```python
from build123d import *

# Parameters (mm, degrees)
SKETCH_2_R          = 2
EXTRUDE_1_DEPTH     = 44.1
CUT_EXTRUDE_START   = -7
CUT_EXTRUDE_1_DEPTH = 7
CHAMFER_1_SIZE      = 0.5
CHAMFER_2_SIZE      = 0.5


with BuildPart() as part:
    # Эскиз2 → Бобышка-Вытянуть1 (new body)
    with BuildSketch(Plane.XY):
        Circle(SKETCH_2_R)
    extrude(amount=EXTRUDE_1_DEPTH)

    # Эскиз3 → Вырез-Вытянуть1 (cut)
    with BuildSketch(Plane.XY.offset(44.1).offset(CUT_EXTRUDE_START)):
        with BuildLine():
            Line((1.322875656, 1.5), (-1.322875656, 1.5))
            ThreePointArc((-1.322875656, 1.5), (0, 2), (1.322875656, 1.5))
        make_face()
    extrude(amount=CUT_EXTRUDE_1_DEPTH, mode=Mode.SUBTRACT)

    # Фаска1
    chamfer_1_edges = [part.edges().sort_by_distance(p)[0] for p in [
        (-2, 0, 0),
    ]]
    chamfer(chamfer_1_edges, length=CHAMFER_1_SIZE)

    # Фаска2
    chamfer_2_edges = [part.edges().sort_by_distance(p)[0] for p in [
        (-0.822875656, -1.822875656, 44.1),
    ]]
    chamfer(chamfer_2_edges, length=CHAMFER_2_SIZE - 0.0001)  # a hair under: the kernel refuses the full size


solid = part.part
```
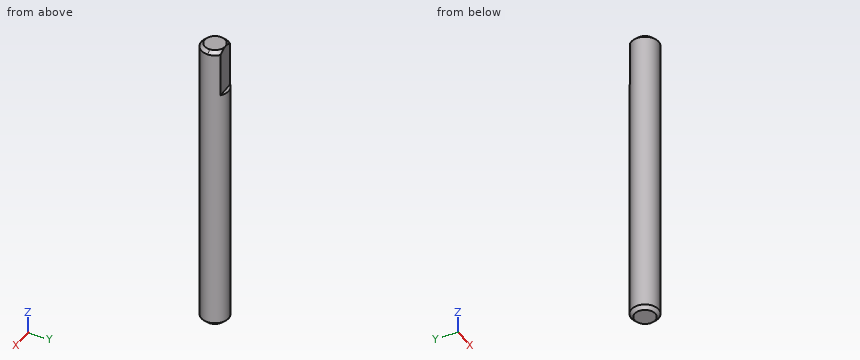
For this review, take the finished solid that the model builds, in its own axes (mm). Coordinates: 2 decimals unless noted, no trailing zeros. Order: outer loops, then holes, each group sorted by start corner. A loop starts at its lowest first (then second) coordinate and runs counter-clockwise, first axis right, second up. Notation, with made-up numbers: (52, 59) - (65, 59) arc R16 ccw to (65, 66) - close; hole circle Ø6 at (23.25, 14). An arc over 180 degrees is marked (long way). Answer as a JSON object with one key per item and string values. Group by question number.
1. For probe 1 along Y at (x, z) = (0.15, 31.5); probe 2 along Y at (x, z) = (1.5, 42); probe 3 along Z at (x, y) = (0.4, 1.6), list the stretches that pass through material, from the lowest coordinate up.
2. Clearance check with flat-ended pins moving along their axes: P1, Ø0.8, axis at x = 0.5, z = 41.5, coming from the +Y side; P2, Ø1, axis at y = -1, z = 21.5, coming from the +X side. State where each tip first meets the part, or that it passes through.
3. We need section A-A on z = 31. State the section outline as (x, y) points, then the cut area to 3 significant figures.
Final values:
{
 "1": {"probe 1": "-1.99 to 1.99", "probe 2": "-1.32 to 1.32", "probe 3": "0.15 to 37.1"},
 "2": {"P1": "y = 1.5", "P2": "x = 1.94"},
 "3": {"outline": "circle Ø4 at (0, 0)", "area": "12.6 mm²"}
}
